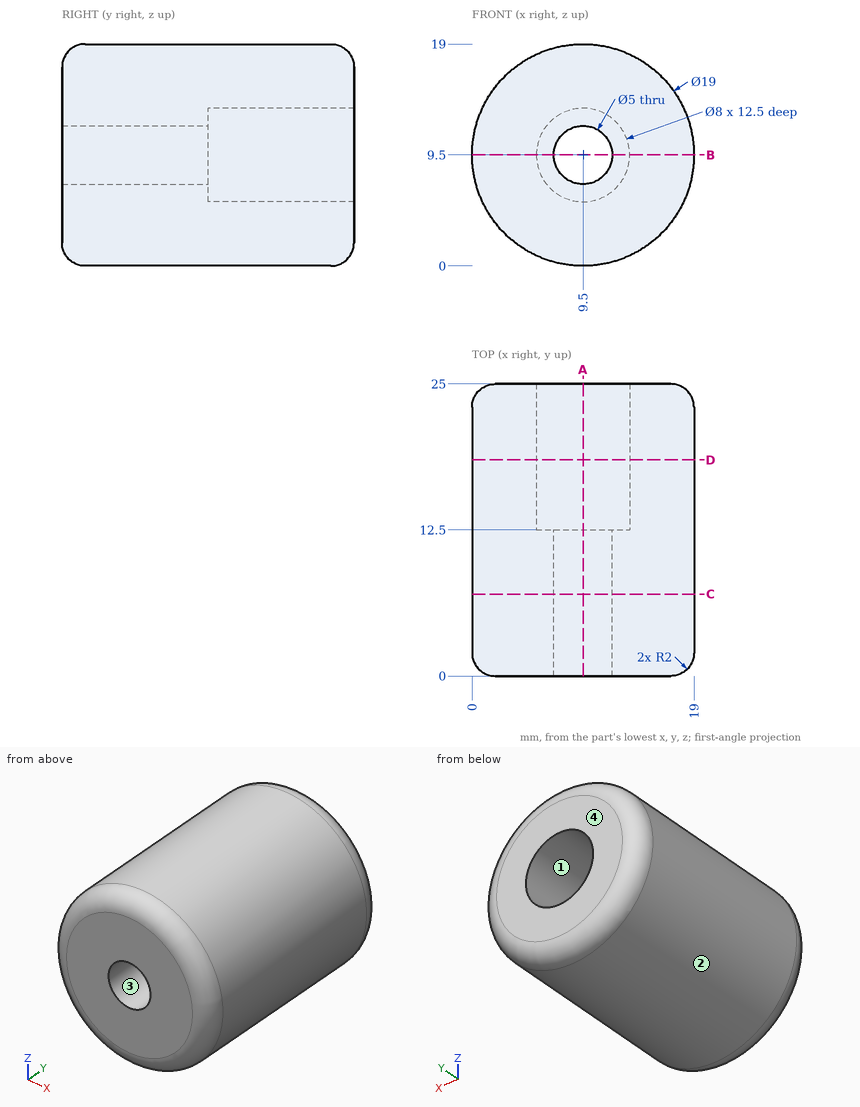
The drawing under review shows one solid part. Ordinate dimensions are in mm from its lowest x, y, z. Give positions to 0.01 mm unless a question says otherwise; leave off trailing zeros. Write each loop counter-clockwise with the first axis right and the second up, starting at its lowest first coordinate (ties: lowest second). Pieces come first, ordered by that corner, then holes. Notation, with made-up numbers: (-13, 10.25) -> (-1, 10.25) arc R24 ccw to (-1, 33.25) -> close; hole circle Ø10 at (59.5, 11). An arc over 180 degrees is marked (long way). Put each result on its own line as item: value.
(1) We need section B-B, the plane z = 9.5. Give the boundary of the cut face in (x, y).
Results are:
outline: (0, 2) arc R2 ccw to (2, 0) -> (7, 0) -> (7, 12.5) -> (5.5, 12.5) -> (5.5, 25) -> (2, 25) arc R2 ccw to (0, 23) -> close; (12, 0) -> (17, 0) arc R2 ccw to (19, 2) -> (19, 23) arc R2 ccw to (17, 25) -> (13.5, 25) -> (13.5, 12.5) -> (12, 12.5) -> close
(2) The part is to be moulded in two halves that separate along X. For the marked faces 1, 2, 3 and 4, say which applies: pulls with the +X half, pulls with the -X half, needs draft (parallel to the pull), parting line crosses it, or undercut.
Results are:
face 1: undercut
face 2: parting line crosses it
face 3: undercut
face 4: needs draft
(3) We need section C-C, the plane y = 7. Give the boundary of the cut face in (x, z).
Results are:
outline: circle Ø19 at (9.5, 9.5); hole circle Ø5 at (9.5, 9.5)
(4) We need section D-D, the plane y = 18.5. Give the boundary of the cut face in (x, z), and give its area (3 significant figures).
Results are:
outline: circle Ø19 at (9.5, 9.5); hole circle Ø8 at (9.5, 9.5)
area: 233 mm²
(5) We need section A-A, the plane x = 9.5. Give the boundary of the cut face in (y, z).
Results are:
outline: (0, 2) arc R2 ccw to (2, 0) -> (23, 0) arc R2 ccw to (25, 2) -> (25, 5.5) -> (12.5, 5.5) -> (12.5, 7) -> (0, 7) -> close; (0, 12) -> (12.5, 12) -> (12.5, 13.5) -> (25, 13.5) -> (25, 17) arc R2 ccw to (23, 19) -> (2, 19) arc R2 ccw to (0, 17) -> close
(6) For pin 1 Ø1 at (y, z) = (3, 11.5) entering from +X; pin 2 Ø7 at (x, z) = (9.5, 9.5) entering from +Y; pin 3 Ø6 at (x, y) = (13.5, 21) entering from -Z, all flat-tipped, find the tip position at first contact; note any pin that passes through.
Results are:
pin 1: x = 18.88
pin 2: y = 12.5
pin 3: z = 0.05
(7) To check wall thickness, follow probe 1 along X at (y, z) = (8, 9.5); probe 2 along Z at (x, y) = (9.25, 20.75); probe 3 along Z at (x, y) = (7.75, 3). State the ranges of each line that lie inside material, in increasing order. Write a range as from..to.
Results are:
probe 1: 0..7, 12..19
probe 2: 0..5.51, 13.49..19
probe 3: 0.16..7.71, 11.29..18.84
